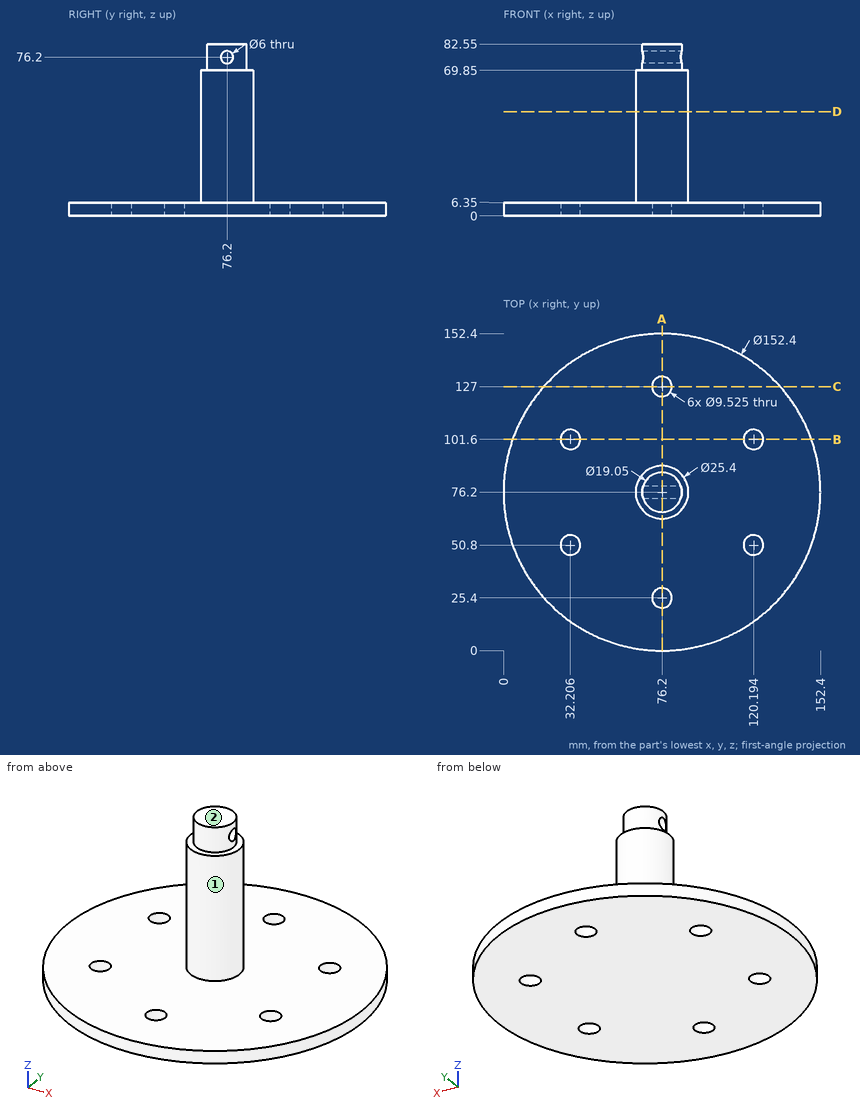
Input: dimensioned drawing with shaded views. Units: mm. Origin: part minimum x, y, z. A direction names the side the tool comes from. Give positions to 0.01 mm unless a question says otherwise; leave off trailing zeros. Order: outer loops, then holes, each group sorted by start corner. A loop starts at its lowest first (then second) coordinate and runs counter-clockwise, first axis right, second up.
(1) Contact query for flat-ended pins moving along their axis: P1, Ø10, axis at y = 70, z = 28.5, coming from the -X side; P2, Ø11, axis at x = 32.21, y = 101.6, coming from the +Z side; P3, Ø2, axis at y = 87.5, z = 14.5, coming from the +X side. Output: stop coordinate, or through.
(2) Section query B-B (y = 101.6). Return the cut outline in (x, z), plus the area to 3 significant figures.
(3) Section query D-D (z = 50). Return the cut outline in (x, y).
(4) Material intervals for line 1 along Y through (x, z) = (76, 2); line 2 along X through (y, z) = (50, 1); line 3 along Z through (x, y) = (22, 61.5), sorted ascending.
(5) Section query C-C (y = 127). Return the cut outline in (x, z).
(6) Access query for the marked faces 1 and 2. Directions: +Z, -Z, +X, -X, +Y, -Y. A direction counts if a zero-diameter tool reaches every point of the face in a straight line with its end or side. Return the directions, or none.
(7) Section query A-A (x = 76.2). State how many separate pieces and enclosed holes the cut face has, plus the area to 3 significant figures.
Outcome:
1. P1: stops at x = 63.56
1. P2: stops at z = 6.35
1. P3: stops at x = 83.63
2. outline: (4.36, 0) - (27.44, 0) - (27.44, 6.35) - (4.36, 6.35) - close; (36.97, 0) - (115.43, 0) - (115.43, 6.35) - (36.97, 6.35) - close; (124.96, 0) - (148.04, 0) - (148.04, 6.35) - (124.96, 6.35) - close
2. area: 791 mm2
3. outline: circle Ø25.4 at (76.2, 76.2)
4. line 1: y = 0 to 20.64, 30.16 to 122.24, 131.76 to 152.4
4. line 2: x = 4.65 to 27.51, 36.9 to 115.5, 124.89 to 147.75
4. line 3: z = 0 to 6.35
5. outline: (19.4, 0) - (71.44, 0) - (71.44, 6.35) - (19.4, 6.35) - close; (80.96, 0) - (133, 0) - (133, 6.35) - (80.96, 6.35) - close
6. face 1: +Z
6. face 2: +Z, +X, -X, +Y, -Y
7. separate pieces: 3
7. enclosed holes: 1
7. area: 2,670 mm2
